Check sheet for the modelled part. Datum: model origin and axes. Units: mm. A direction names the side the tool comes from. Give positions to 0.01 mm unless a question says otherwise; leave off trailing zeros. Loops run counter-clockwise (first coordinate to the right, second up) from the corner with the lowest first, then second, coordinate; pieces in that order, holes last. Notation, with made-up numbers: (39, 27.25) -> (98, 27.25) arc R16 ccw to (98, 37.25) -> close; hole circle Ø7 at (-29.5, -36.5). An arc over 180 degrees is marked (long way). Answer as CSV lines item,"result". Start each with the question number.
(1) Access from +Z, -Z, +X, -X, +Y, -Y to the whole of each face (thin tool, end or side, straight path). Record for faces 1 (the face through (-11.2, -7.4, 0.1)), 2 (the face through (-4, -2, -2.75)).
(2) Section check B-B on y = -2.25. Enter the section's corners in (x, z).
(3) Release check for a two-part mould opening along X. For faces 3 (the face through (-0.509, -3.991, -2.294)), 4 (the face through (-11.65, -3.89, 0.08)) record: pulls with the +X half, pulls with the -X half, needs draft (parallel to the pull), parting line crosses it, or undercut.
(4) Section check C-C on y = -7.5. Enter the section's corners in (x, z).
(5) Section check A-A on x = 0. Enter the section's corners in (y, z), plus the area to 3 significant figures.
(6) Section check D-D on x = -7.5. Enter the section's corners in (y, z).
(7) Material ranges on line 1 (Z direction, x = 8, y = -5.15); line 2 (X direction, y = -2.25, z = 1.5); line 3 (Z direction, x = -4.25, y = -0.75), recorded low to high. Write a range as from..to.
(8) Gauge pin test, flat ends, axial feed: pin 1 Ø2 at (x, z) = (-0.5, -1.5) entering from -Y; pin 2 Ø1 at (x, z) = (-2, -0.5) entering from +Y; pin 3 Ø3 at (y, z) = (-1.5, 2) entering from +X. Record the tip position at first contact, or that the pin passes through.
from build123d import *

# Parameters (mm, degrees)
F1_DEPTH  = 7.9
F2_R      = 3.2
F2_R_2    = 2.35
F3_DEPTH  = 1
F3_FACE_R = 2.35
F4_R      = 2.35
F5_DEPTH  = 7.901
F6_R      = 3.2
F6_R_2    = 2.35
F7_DEPTH  = 1
F9_DEPTH  = 3.6
F11_DEPTH = 3.6
F12_R     = 0.3


with BuildPart() as f1:
    # F0 (on Front) → F1 (new body)
    with BuildSketch(Plane.XZ):
        with BuildLine():
            Line((-8, -3.65), (8, -3.65))
            ThreePointArc((8, -3.65), (11.65, 0), (8, 3.65))
            Line((8, 3.65), (-8, 3.65))
            ThreePointArc((-8, 3.65), (-11.65, 0), (-8, -3.65))
        make_face()
    extrude(amount=F1_DEPTH)

    # F2 (on face) → F3 (cut)
    with BuildSketch(Plane.XZ.offset(7.9)):
        with Locations((-8, 0)):
            Circle(F2_R)
        with Locations((-8, 0)):
            Circle(F2_R_2, mode=Mode.SUBTRACT)
        Circle(F2_R)
        Circle(F2_R_2, mode=Mode.SUBTRACT)
        with Locations((8, 0)):
            Circle(F2_R)
        with Locations((8, 0)):
            Circle(F2_R_2, mode=Mode.SUBTRACT)
    extrude(amount=-F3_DEPTH, mode=Mode.SUBTRACT)

    # F3_face (on face) + F4 (on face) → F5 (cut, through all)
    with BuildSketch(Plane.XZ.offset(7.9)):
        with Locations((-8, 0)):
            Circle(F3_FACE_R)
        with Locations((8, 0)):
            Circle(F3_FACE_R)
    with BuildSketch(Plane.XZ.offset(7.9)):
        Circle(F4_R)
    extrude(amount=-F5_DEPTH, mode=Mode.SUBTRACT)

    # F6 (on face) → F7 (cut)
    with BuildSketch(Plane(origin=(0, 0, 0), x_dir=(-1, 0, 0), z_dir=(0, 1, 0))):
        with Locations((8, 0)):
            Circle(F6_R)
        with Locations((8, 0)):
            Circle(F6_R_2, mode=Mode.SUBTRACT)
        Circle(F6_R)
        Circle(F6_R_2, mode=Mode.SUBTRACT)
        with Locations((-8, 0)):
            Circle(F6_R)
        with Locations((-8, 0)):
            Circle(F6_R_2, mode=Mode.SUBTRACT)
    extrude(amount=-F7_DEPTH, mode=Mode.SUBTRACT)

    # F8 (on face) → F9 (cut)
    with BuildSketch(Plane.XZ.offset(7.9)):
        with BuildLine():
            ThreePointArc((5.6, -2.75), (4.35, 0), (5.6, 2.75))
            Line((5.6, 2.75), (2.4, 2.75))
            ThreePointArc((2.4, 2.75), (3.3228376427, 1.5103807467), (3.65, 0))
            ThreePointArc((3.65, 0), (3.3228376427, -1.5103807467), (2.4, -2.75))
            Line((2.4, -2.75), (5.6, -2.75))
        make_face()
        with BuildLine():
            ThreePointArc((-2.4, -2.75), (-3.65, 0), (-2.4, 2.75))
            Line((-2.4, 2.75), (-5.6, 2.75))
            ThreePointArc((-5.6, 2.75), (-4.6771623573, 1.5103807467), (-4.35, 0))
            ThreePointArc((-4.35, 0), (-4.6771623573, -1.5103807467), (-5.6, -2.75))
            Line((-5.6, -2.75), (-2.4, -2.75))
        make_face()
    extrude(amount=-F9_DEPTH, mode=Mode.SUBTRACT)

    # F10 (on face) → F11 (cut)
    with BuildSketch(Plane(origin=(0, 0, 0), x_dir=(-1, 0, 0), z_dir=(0, 1, 0))):
        with BuildLine():
            ThreePointArc((5.6, -2.75), (4.35, 0), (5.6, 2.75))
            Line((5.6, 2.75), (2.4, 2.75))
            ThreePointArc((2.4, 2.75), (3.3228376427, 1.5103807467), (3.65, 0))
            ThreePointArc((3.65, 0), (3.3228376427, -1.5103807467), (2.4, -2.75))
            Line((2.4, -2.75), (5.6, -2.75))
        make_face()
        with BuildLine():
            ThreePointArc((-2.4, -2.75), (-3.65, 0), (-2.4, 2.75))
            Line((-2.4, 2.75), (-5.6, 2.75))
            ThreePointArc((-5.6, 2.75), (-4.6771623573, 1.5103807467), (-4.35, 0))
            ThreePointArc((-4.35, 0), (-4.6771623573, -1.5103807467), (-5.6, -2.75))
            Line((-5.6, -2.75), (-2.4, -2.75))
        make_face()
    extrude(amount=-F11_DEPTH, mode=Mode.SUBTRACT)

    # F12
    f12_edges = [f1.edges().sort_by_distance(p)[0] for p in [
        (-5.6, -1.8, 2.75),
        (2.4, -1.8, 2.75),
        (2.4, -6.1, 2.75),
        (-5.6, -6.1, 2.75),
        (-2.4, -6.1, 2.75),
        (5.6, -6.1, 2.75),
        (-2.4, -1.8, 2.75),
        (5.6, -1.8, 2.75),
        (-5.6, -1.8, -2.75),
        (2.4, -1.8, -2.75),
        (-2.4, -1.8, -2.75),
        (5.6, -1.8, -2.75),
        (-2.4, -6.1, -2.75),
        (5.6, -6.1, -2.75),
        (-5.6, -6.1, -2.75),
        (2.4, -6.1, -2.75),
    ]]
    fillet(f12_edges, radius=F12_R)


solid = f1.part
Working result:
1,face 1,"-Y"
1,face 2,"+Y"
2,outline,"(-8, -3.65) -> (8, -3.65) arc R3.65 ccw to (8, 3.65) -> (-8, 3.65) arc R3.65 ccw to start; hole circle Ø4.7 at (-8, 0); hole (-5.14, -2.26) arc R0.3 ccw to (-4.9, -2.75) -> (-3.1, -2.75) arc R0.3 ccw to (-2.86, -2.26) arc R3.65 cw to (-2.86, 2.26) arc R0.3 ccw to (-3.1, 2.75) -> (-4.9, 2.75) arc R0.3 ccw to (-5.14, 2.26) arc R3.65 cw to start; hole circle Ø4.7 at (0, 0); hole (2.86, -2.26) arc R0.3 ccw to (3.1, -2.75) -> (4.9, -2.75) arc R0.3 ccw to (5.14, -2.26) arc R3.65 cw to (5.14, 2.26) arc R0.3 ccw to (4.9, 2.75) -> (3.1, 2.75) arc R0.3 ccw to (2.86, 2.26) arc R3.65 cw to start; hole circle Ø4.7 at (8, 0)"
3,face 3,"undercut"
3,face 4,"pulls with the -X half"
4,outline,"(-8, -3.65) -> (8, -3.65) arc R3.65 ccw to (8, 3.65) -> (-8, 3.65) arc R3.65 ccw to start; hole circle Ø6.4 at (-8, 0); hole (-5.14, -2.26) arc R0.3 ccw to (-4.9, -2.75) -> (-3.1, -2.75) arc R0.3 ccw to (-2.86, -2.26) arc R3.65 cw to (-2.86, 2.26) arc R0.3 ccw to (-3.1, 2.75) -> (-4.9, 2.75) arc R0.3 ccw to (-5.14, 2.26) arc R3.65 cw to start; hole circle Ø6.4 at (0, 0); hole (2.86, -2.26) arc R0.3 ccw to (3.1, -2.75) -> (4.9, -2.75) arc R0.3 ccw to (5.14, -2.26) arc R3.65 cw to (5.14, 2.26) arc R0.3 ccw to (4.9, 2.75) -> (3.1, 2.75) arc R0.3 ccw to (2.86, 2.26) arc R3.65 cw to start; hole circle Ø6.4 at (8, 0)"
5,outline,"(-7.9, -3.65) -> (0, -3.65) -> (0, -3.2) -> (-1, -3.2) -> (-1, -2.35) -> (-6.9, -2.35) -> (-6.9, -3.2) -> (-7.9, -3.2) -> close; (-7.9, 3.2) -> (-6.9, 3.2) -> (-6.9, 2.35) -> (-1, 2.35) -> (-1, 3.2) -> (0, 3.2) -> (0, 3.65) -> (-7.9, 3.65) -> close"
5,area,"17.1 mm^2"
6,outline,"(-7.9, -3.65) -> (0, -3.65) -> (0, -3.16) -> (-1, -3.16) -> (-1, -2.3) -> (-6.9, -2.3) -> (-6.9, -3.16) -> (-7.9, -3.16) -> close; (-7.9, 3.16) -> (-6.9, 3.16) -> (-6.9, 2.3) -> (-1, 2.3) -> (-1, 3.16) -> (0, 3.16) -> (0, 3.65) -> (-7.9, 3.65) -> close"
7,line 1,"z = -3.65..-2.35, 2.35..3.65"
7,line 2,"x = -11.33..-9.81, -6.19..-4.67, -3.33..-1.81, 1.81..3.33, 4.67..6.19, 9.81..11.33"
7,line 3,"z = -3.65..-2.75, 2.75..3.65"
8,pin 1,"stops at y = -6.9"
8,pin 2,"stops at y = -1"
8,pin 3,"stops at x = 11.62"
